from build123d import *

# Parameters (mm, degrees)
BOSS_EXTRU_1_DEPTH = 250
CONG_1_R           = 55
CONG_2_R           = 2


with BuildPart() as part:
    # Esquisse1 → Boss.-Extru.1 (new body)
    with BuildSketch(Plane.XY):
        with BuildLine():
            Line((0, 0), (55, 0))
            Line((55, 0), (55, -20))
            Line((55, -20), (150, -20))
            Line((150, -20), (150, -10))
            ThreePointArc((150, -10), (185, 25), (220, -10))
            Line((220, -10), (220, -20))
            Line((220, -20), (250, -20))
            Line((250, -20), (250, 35))
            Line((250, 35), (184.403047163, 35))
            ThreePointArc((184.403047163, 35), (155.280415441, 24.305572748), (140, -2.694563485))
            Line((140, -2.694563485), (140, -11))
            Line((140, -11), (65, -15))
            Line((65, -15), (65, 5))
            Line((65, 5), (0, 5))
            Line((0, 5), (0, 0))
        make_face()
    extrude(amount=BOSS_EXTRU_1_DEPTH)

    # Congé1
    cong_1_edges = [part.edges().sort_by_distance(p)[0] for p in [
        (0, 2.5, 0),
        (0, 2.5, 250),
    ]]
    fillet(cong_1_edges, radius=CONG_1_R)

    # Congé2
    cong_2_edges = [part.edges().sort_by_distance(p)[0] for p in [
        (65, 5, 125),
    ]]
    fillet(cong_2_edges, radius=CONG_2_R)


solid = part.part
Can you work these out from the model? Positions are in its coordinate system, mm. A direction names the side the tool comes from. Round coordinates to 2 decimals unless told otherwise and drop trailing zeros. Order: outer loops, then holes, each group sorted by start corner. A loop starts at its lowest first (then second) coordinate and runs counter-clockwise, first axis right, second up. Notation, with made-up numbers: (23, 69) - (46, 69) arc R13 cw to (46, 79) - close; hole circle Ø2 at (89.5, -6). An arc over 180 degrees is marked (long way). Answer in a Markdown table with one row per item.
(1) Suppose I cut it at D-D, the plane z = 230.5. Please give me the cut outline in (x, y).
From the geometry:
| item | result |
|---|---|
| outline | (12.99, 0) - (55, 0) - (55, -20) - (150, -20) - (150, -10) arc R35 cw to (220, -10) - (220, -20) - (250, -20) - (250, 35) - (184.4, 35) arc R45 ccw to (140, -2.69) - (140, -11) - (65, -15) - (65, 3) arc R2 ccw to (63, 5) - (12.99, 5) - close |
(2) Suppose I cut it at B-B, the plane y = 20. Please give me the cut outline in (x, z).
From the geometry:
| item | result |
|---|---|
| outline | (150.86, 0) - (166.97, 0) - (166.97, 250) - (150.86, 250) - close; (203.03, 0) - (250, 0) - (250, 250) - (203.03, 250) - close |
(3) Suppose I cut it at A-A, the plane z = 112.5. Please give me the cut outline in (x, y).
From the geometry:
| item | result |
|---|---|
| outline | (0, 0) - (55, 0) - (55, -20) - (150, -20) - (150, -10) arc R35 cw to (220, -10) - (220, -20) - (250, -20) - (250, 35) - (184.4, 35) arc R45 ccw to (140, -2.69) - (140, -11) - (65, -15) - (65, 3) arc R2 ccw to (63, 5) - (0, 5) - close |
(4) If we mould it in two halves opening along X, with no side actions, what happens to faces 4 (the face through (218, 35, 123)), 5 (the face through (55, -10, 123)), 6 (the face through (140, -7, 123))? For each: released by +X, released by -X, zero draft, split by the parting line, or undercut.
From the geometry:
| item | result |
|---|---|
| face 4 | zero draft |
| face 5 | released by -X |
| face 6 | undercut |
(5) Which directions (+Z, -Z, +X, -X, +Y, -Y) give clear straight access to the entire face, cutting with the end or side of a thin tool? Please do faces 1 (the face through (27, 0, 123)), 2 (the face through (103.025, -12.972, 123.25)), 3 (the face through (150, -15, 123)).
From the geometry:
| item | result |
|---|---|
| face 1 | +Z, -Z, -X, -Y |
| face 2 | +Z, -Z, +Y |
| face 3 | +Z, -Z, -Y |
(6) For P1, Ø12, axis at x = 169.5, z = 220, coming from the -Y side; P2, Ø3, axis at y = -13, z = 137, coming from the -X side; P3, Ø16.5, axis at x = 17, z = 136.5, coming from the -Y side, each with a flat end and sliding along its axis, tell me the tip position at first contact or that it passes through.
From the geometry:
| item | result |
|---|---|
| P1 | stops at y = 17.62 |
| P2 | stops at x = 55 |
| P3 | stops at y = 0 |
(7) Please list where these lines run through material, in increasing order: L1, parallel to X at y = -8, z = 136; L2, parallel to X at y = -3, z = 138; L3, parallel to Y at x = 43, z = 59.5. Write a range as from..to.
From the geometry:
| item | result |
|---|---|
| L1 | x = 55..65, 140..150.06, 219.94..250 |
| L2 | x = 55..65, 140..150.71, 219.29..250 |
| L3 | y = 0..5 |
(8) Suppose I cut it at C-C, the plane x = 131. Please give me the cut outline in (y, z), plus the area to 3 significant figures.
From the geometry:
| item | result |
|---|---|
| outline | (-20, 0) - (-11.48, 0) - (-11.48, 250) - (-20, 250) - close |
| area | 2,130 mm2 |
